Part print with two shaded views. Sizes in mm from the minimum x, y, z corner. Coordinates: 2 decimals unless noted, no trailing zeros. Write each loop counter-clockwise with the first axis right and the second up, starting at its lowest first coordinate (ties: lowest second). Pieces come first, ordered by that corner, then holes.
Q1. Drill centre lines: probe 1 along Y at (x, z) = (23, 176); probe 2 along Y at (x, z) = (17, 224.5); probe 3 along X at (y, z) = (34, 194.5). Where is each one in solid material? Low to high.
Q2. Pin check, flat tips, straight feed: P1, Ø6, axis at x = 15.5, y = 18.5, coming from the +Z side; P2, Ø1.5, axis at x = 19, y = 10.5, coming from the -Z side; P3, Ø1.5, axis at x = 18, z = 198, coming from the +Y side. Stop position of each tip, or through.
Q3. Band-saw the part on B-B, the plane z = 204. Write the cut outline in (x, y), plus the area to 3 significant figures.
Q4. Band-saw the part on A-A, the plane y = 13. Write the cut outline in (x, z), plus the area to 3 significant figures.
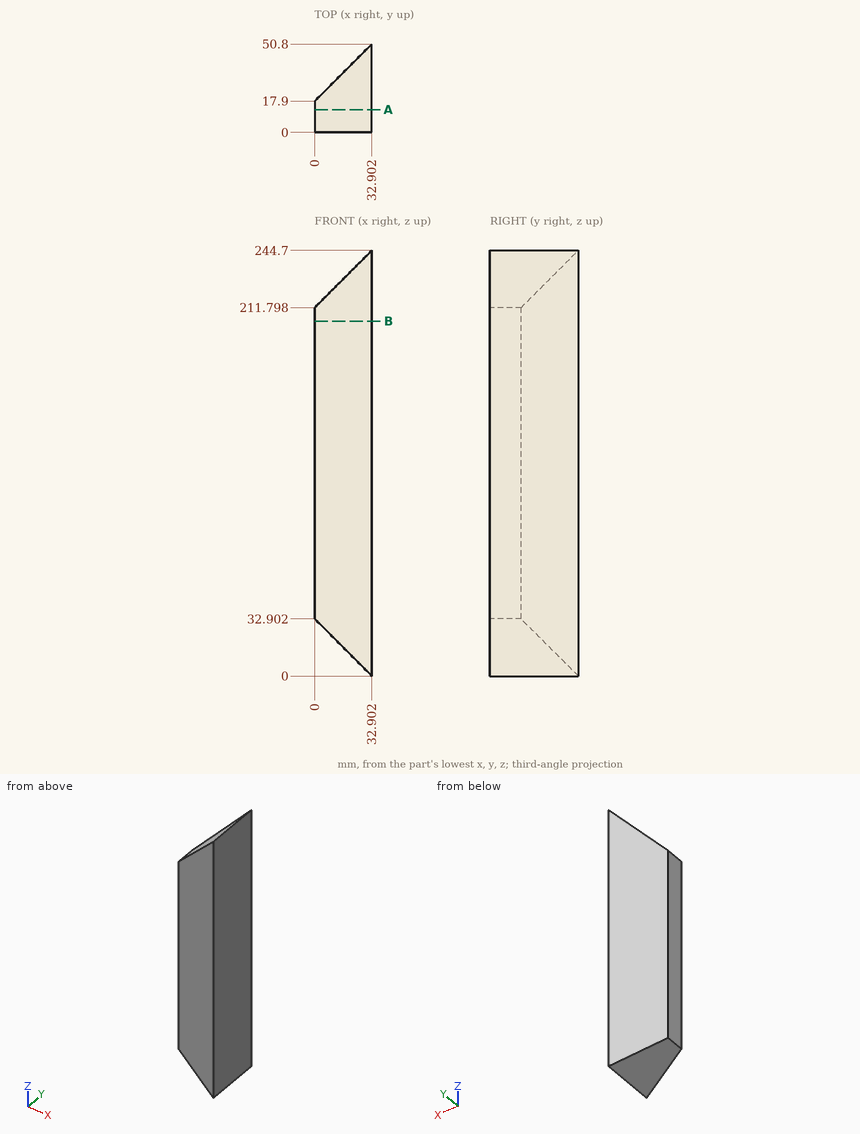
Answer sheet:
1. probe 1: y = 0 to 40.9
1. probe 2: y = 0 to 34.9
1. probe 3: x = 16.1 to 32.9
2. P1: stops at z = 230.3
2. P2: stops at z = 13.15
2. P3: stops at y = 36.65
3. outline: (0, 0) - (32.9, 0) - (32.9, 50.8) - (0, 17.9) - close
3. area: 1,130 mm2
4. outline: (0, 32.9) - (32.9, 0) - (32.9, 244.7) - (0, 211.8) - close
4. area: 6,970 mm2
